Design review of the part built by this model. Coordinates are the model's own, in mm. A direction names the side the tool comes from. Give positions to 0.01 mm unless a question says otherwise; leave off trailing zeros. Put each result on its own line as item: value. Start each with the question number.
from build123d import *

# Parameters (mm, degrees)
F0_W     = 0.6
F0_H     = 8
F1_DEPTH = 15
F2_SIZE  = 1
F3_W     = 0.85
F3_H     = 15.628527
F4_DEPTH = 25
F5_W     = 0.5
F5_H     = 8
F6_DEPTH = 10


with BuildPart() as f1:
    # F0 (on Top) → F1 (new body)
    with BuildSketch(Plane.XY):
        with BuildLine():
            Line((0, -4), (0, 15))
            ThreePointArc((0, 15), (-15, 0), (0, -15))
            Line((0, -15), (0, -12))
            Line((0, -12), (-0.6, -12))
            Line((-0.6, -12), (-0.6, -4))
            Line((-0.6, -4), (0, -4))
        make_face()
        with Locations((-0.3, -8)):
            Rectangle(F0_W, F0_H)
    extrude(amount=F1_DEPTH)

    # F2
    f2_edges = [f1.edges().sort_by_distance(p)[0] for p in [
        (-15, 0, 15),
        (-15, 0, 0),
    ]]
    chamfer(f2_edges, length=F2_SIZE)

    # F3 (on face) → F4 (cut)
    with BuildSketch(Plane.XY.offset(15)):
        with Locations((-0.425, -7.814656)):
            Rectangle(F3_W, F3_H)
    extrude(amount=-F4_DEPTH, mode=Mode.SUBTRACT)

    # F5 (on face) → F6 (cut)
    with BuildSketch(Plane.XY.offset(15)):
        with Locations((-1.1, -8.000393)):
            Rectangle(F5_W, F5_H)
    extrude(amount=-F6_DEPTH, mode=Mode.SUBTRACT)


solid = f1.part
1. Machinability: for faces 1 (the flat face through (-0.85, -8, 4)), 2 (the flat face through (0, 7, 7)), which of the approach directions +Z, -Z, +X, -X, +Y, -Y give a long, thin tool a straight path to every point of the face, cutting with its end or side? Answer none if there is none.
2. The part is to be moulded in two halves that separate along Y. For faces 3 (the flat face through (-6, 0, 15)), 4 (the flat face through (-0.4, 0, 7.6)), 5 (the cylindrical face through (-14.98, 0.75, 7.41)), 6 (the flat face through (-1.35, -8, 10)), say which applies: +Y half, -Y half, draft (parallel to the pull), parting line (faces both ways), or undercut.
3. To check wall thickness, follow probe 1 along X at (y, z) = (7, 1.75); probe 2 along Y at (x, z) = (-5.5, 7.5); probe 3 along Y at (x, z) = (-9, 8). State the ranges of each line that lie inside material, in increasing order.
4. Insertion check: pin 1 (8 mm diameter, centred on x = -10, z = 6, fed in from -Y); pin 2 (6 mm diameter, centred on x = -5, z = 6.5, fed in from +Y); pin 3 (6.5 mm diameter, centred on y = -6.5, z = 8.5, fed in from +X). Each pin has a flat end and moves straight along its axis. Give the tip position at first contact, or say it passes through.
Returned:
1. face 1: +Z, -Z, +X, -Y
1. face 2: +Z, -Z, +X, +Y, -Y
2. face 3: draft
2. face 4: -Y half
2. face 5: parting line
2. face 6: undercut
3. probe 1: x = -13.27 to 0
3. probe 2: y = -13.96 to 13.96
3. probe 3: y = -12 to 12
4. pin 1: stops at y = -13.75
4. pin 2: stops at y = 14.87
4. pin 3: stops at x = -0.85
